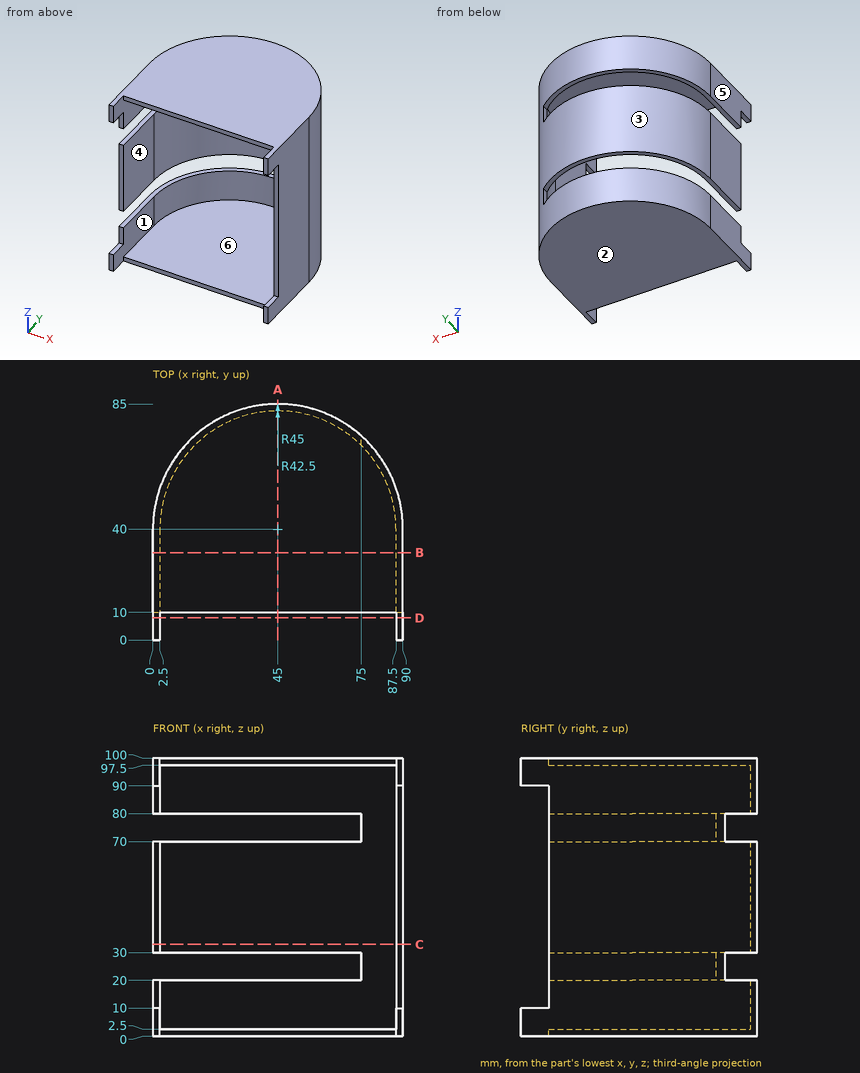
Geometry: see drawing. Coordinates: mm, zero at the bounding-box minimum. A direction names the side the tool comes from. Give positions to 0.01 mm unless a question says otherwise; leave off trailing zeros. Loops run counter-clockwise (first coordinate to the right, second up) from the corner with the lowest first, then second, coordinate; pieces in that order, holes last. Notation, with made-up numbers: (31, 42.5) -> (52, 42.5) arc R11 ccw to (52, 56.5) -> close; hole circle Ø11 at (20.5, -26.75). An arc over 180 degrees is marked (long way). Answer as a JSON object with one key per item and string values. Group by question number.
Item 1: Cut plane B-B, the plane y = 31.5. Return the cut outline in (x, z).
Item 2: Cut plane C-C, the plane z = 33. Return the cut outline in (x, y).
Item 3: Line query: probe 1 along Z at (x, y) = (9.5, 66); probe 2 along Z at (x, y) = (53, 14); probe 3 along X at (y, z) = (18.5, 31). Output: solid intervals per line, ascending.
Item 4: Cut plane D-D, the plane y = 8. Return the cut outline in (x, z).
Item 5: Pin query (flat end, axial travel): P1, Ø0.8, axis at x = 1.5, z = 86.5, coming from the -Y side; P2, Ø1, axis at x = 13, z = 12, coming from the -Y side; P3, Ø1, axis at x = 13, z = 37, coming from the +Y side. Return the tip coordinate at first contact, or that it passes through.
Item 6: Cut plane A-A, the plane x = 45. Return the cut outline in (y, z), and give its area (4 significant figures).
Item 7: Reachability of the marked faces 5 and 6 from +Z, -Z, +X, -X, +Y, -Y: full face, straight path, thin tool, end or side. Return the list, or none.
Item 8: Pull-direction query (X, two-part tool) for the marked faces 1, 2, 3 and 4; classes: released by +X, released by -X, zero draft, split by the parting line, or undercut.
Checks:
{
 "1": {"outline": "(0, 0) -> (90, 0) -> (90, 100) -> (0, 100) -> (0, 80) -> (2.5, 80) -> (2.5, 97.5) -> (87.5, 97.5) -> (87.5, 2.5) -> (2.5, 2.5) -> (2.5, 20) -> (0, 20) -> close; (0, 30) -> (2.5, 30) -> (2.5, 70) -> (0, 70) -> close"},
 "2": {"outline": "(0, 10) -> (2.5, 10) -> (2.5, 40) arc R42.5 cw to (87.5, 40) -> (87.5, 10) -> (90, 10) -> (90, 40) arc R45 ccw to (0, 40) -> close"},
 "3": {"probe 1": "z = 0 to 20, 30 to 70, 80 to 100", "probe 2": "z = 0 to 2.5, 97.5 to 100", "probe 3": "x = 0 to 2.5, 87.5 to 90"},
 "4": {"outline": "(0, 0) -> (2.5, 0) -> (2.5, 10) -> (0, 10) -> close; (0, 90) -> (2.5, 90) -> (2.5, 100) -> (0, 100) -> close; (87.5, 0) -> (90, 0) -> (90, 10) -> (87.5, 10) -> close; (87.5, 90) -> (90, 90) -> (90, 100) -> (87.5, 100) -> close"},
 "5": {"P1": "stops at y = 10", "P2": "stops at y = 67.39", "P3": "stops at y = 72.14"},
 "6": {"outline": "(10, 0) -> (85, 0) -> (85, 20) -> (82.5, 20) -> (82.5, 2.5) -> (10, 2.5) -> close; (10, 97.5) -> (82.5, 97.5) -> (82.5, 80) -> (85, 80) -> (85, 100) -> (10, 100) -> close; (82.5, 30) -> (85, 30) -> (85, 70) -> (82.5, 70) -> close", "area": "562.5 mm²"},
 "7": {"face 5": "+Z, -Z, -X, +Y, -Y", "face 6": "-Y"},
 "8": {"face 1": "undercut", "face 2": "zero draft", "face 3": "split by the parting line", "face 4": "undercut"}
}
